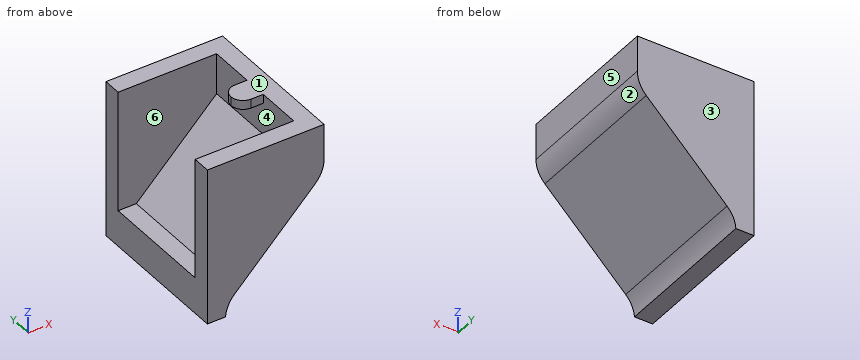
```python
from build123d import *

# Parameters (mm, degrees)
SKETCH_1_W          = 10
SKETCH_1_H          = 15
EXTRUDE_1_DEPTH     = 3
SKETCH_2_W          = 3
SKETCH_2_H          = 25
EXTRUDE_2_DEPTH     = 6
EXTRUDE_3_DEPTH     = 25
EXTRUDE_4_DEPTH     = 3
EXTRUDE_5_DEPTH     = 3
FILLET_1_R          = 5
SKETCH_6_W          = 10
SKETCH_6_H          = 15
CUT_EXTRUDE_1_DEPTH = 3
FILLET_2_R          = 5
SKETCH_7_W          = 1.5
SKETCH_7_H          = 4
EXTRUDE_6_DEPTH     = 4
FILLET_3_R          = 2


# Some blends are built 0.0001 mm under size
with BuildPart() as part:
    # 草图1 → 凸台-拉伸1 (new body)
    with BuildSketch(Plane.XY):
        with Locations((5, -7.5)):
            Rectangle(SKETCH_1_W, SKETCH_1_H)
    extrude(amount=EXTRUDE_1_DEPTH)

    # 草图2 → 凸台-拉伸2 (add)
    with BuildSketch(Plane.XY.offset(3)):
        with Locations((8.5, -7.5)):
            Rectangle(SKETCH_2_W, SKETCH_2_H)
    extrude(amount=EXTRUDE_2_DEPTH)

    # 草图3 → 凸台-拉伸3 (add)
    with BuildSketch(Plane(origin=(0, -20, 0), x_dir=(-1, 0, 0), z_dir=(0, -1, 0))):
        Polygon((-10, -9), (-23.263455967, -22.263455967), (-23.263455967, -29.02081528), (-26.263455967, -29.02081528), (-26.263455967, -21.02081528), (-10, -4.757359313), align=None)
    extrude(amount=-EXTRUDE_3_DEPTH)

    # 草图4 → 凸台-拉伸4 (add)
    with BuildSketch(Plane(origin=(0, -20, 0), x_dir=(-1, 0, 0), z_dir=(0, -1, 0))):
        Polygon((-7, -9), (-10, -9), (-23.263455967, -22.263455967), (-23.263455967, -29.02081528), (-7, -29.02081528), align=None)
    extrude(amount=-EXTRUDE_4_DEPTH)

    # 草图5 → 凸台-拉伸5 (add)
    with BuildSketch(Plane(origin=(0, 5, 0), x_dir=(1, 0, 0), z_dir=(0, 1, 0))):
        Polygon((7, -9), (10, -9), (23.263455967, -22.263455967), (23.263455967, -29.02081528), (7, -29.02081528), align=None)
    extrude(amount=-EXTRUDE_5_DEPTH)

    # 圆角1
    fillet_1_edges = [part.edges().sort_by_distance(p)[0] for p in [
        (26.263455967, -7.5, 21.02081528),
    ]]
    fillet(fillet_1_edges, radius=FILLET_1_R)

    # 草图6 → 切除-拉伸1 (cut)
    with BuildSketch(Plane(origin=(0, 0, 0), x_dir=(-1, 0, 0), z_dir=(0, 0, -1))):
        with Locations((-5, -7.5)):
            Rectangle(SKETCH_6_W, SKETCH_6_H)
    extrude(amount=-CUT_EXTRUDE_1_DEPTH, mode=Mode.SUBTRACT)

    # 圆角2
    # the kernel refuses this fillet: 5 mm, written as the material it adds along each edge
    with BuildSketch(Plane(origin=(10, -20, 4.757359313), x_dir=(0, 0, -1), z_dir=(0, 1, 0))) as fillet_2_piece_1:
        with BuildLine():
            CenterArc((2.08159154, -4.989476271), FILLET_2_R, 93.718036518, 41.281963482)
            Line((-1.453942365, -1.453942365), (-1.524653044, -1.383231687))
            Line((-1.524653044, -1.383231687), (-0.070710678, 0.070710678))
            Line((-0.070710678, 0.070710678), (0, 0.1))
            ThreePointArc((0, 0.1), (0.878679656, 0.1), (1.750874668, 0.099789525))
            Line((1.750874668, 0.099789525), (1.757359313, 0))
        make_face()
    extrude(amount=25)

    # 草图7 → 凸台-拉伸6 (add)
    with BuildSketch(Plane.ZY.offset(-23.263455967)):
        with Locations((28.27081528, -7.5)):
            Rectangle(SKETCH_7_W, SKETCH_7_H)
    extrude(amount=EXTRUDE_6_DEPTH)

    # 圆角3
    fillet_3_edges = [part.edges().sort_by_distance(p)[0] for p in [
        (19.263455967, -9.5, 28.27081528),
        (19.263455967, -5.5, 28.27081528),
    ]]
    fillet(fillet_3_edges, radius=FILLET_3_R - 0.0001)  # a hair under: the kernel refuses the full size


solid = part.part
```
Read the model definition and answer for the solid it produces. Units are mm, in the model's axes. Face numbers are marked on the shaded views. A direction names the side the tool comes from. Give positions to 0.01 mm unless a question says otherwise; leave off trailing zeros. Order: outer loops, then holes, each group sorted by start corner. A loop starts at its lowest first (then second) coordinate and runs counter-clockwise, first axis right, second up. Notation, with made-up numbers: (65, 50) -> (81, 50) arc R32 cw to (81, 77) -> close; hole circle Ø3 at (-39, -29.75). An arc over 180 degrees is marked (long way). Write item = value, one per line.
1. A cutting plane is placed at A-A, the plane x = 9. Write down the section's boundary in (y, z).
Numbers:
outline = (-20, 3) -> (5, 3) -> (5, 29.02) -> (2, 29.02) -> (2, 9) -> (-17, 9) -> (-17, 29.02) -> (-20, 29.02) -> close
2. For the marked faces 5 and 6, determine the directions among +Z, -Z, +X, -X, +Y, -Y from which every point of the face is accessible in a straight line to the end or side of a thin tool.
Numbers:
face_5 = +Z, -Z, +X, +Y, -Y
face_6 = +Z, -X
3. Straight lines are drawn through the part: line 1 along Y through (x, z) = (18.75, 20.75); line 2 along X through (y, z) = (-11.75, 27); line 3 along X through (y, z) = (-15, 20.5). For each, find the intervals that lie inside material, in ascending order.
Numbers:
line_1 = -20 to -17, 2 to 5
line_2 = 23.26 to 26.26
line_3 = 21.5 to 25.54
4. A cutting plane is placed at D-D, the plane z = 18.5. Write down the section's boundary in (x, y).
Numbers:
outline = (7, -20) -> (23.74, -20) -> (23.74, 5) -> (7, 5) -> (7, 2) -> (19.5, 2) -> (19.5, -17) -> (7, -17) -> close
5. A cutting plane is placed at C-C, the plane x = 22.5. Write down the section's boundary in (y, z).
Numbers:
outline = (-20, 17.26) -> (5, 17.26) -> (5, 29.02) -> (2, 29.02) -> (2, 21.5) -> (-17, 21.5) -> (-17, 29.02) -> (-20, 29.02) -> close; (-9.5, 27.52) -> (-5.5, 27.52) -> (-5.5, 29.02) -> (-9.5, 29.02) -> close
6. A cutting plane is placed at B-B, the plane y = -10. Write down the section's boundary in (x, z).
Numbers:
outline = (7, 3) -> (10, 3) arc R5 cw to (11.45, 6.21) -> (24.8, 19.56) arc R5 ccw to (26.26, 23.09) -> (26.26, 29.02) -> (23.26, 29.02) -> (23.26, 22.26) -> (10, 9) -> (7, 9) -> close
7. Given pin 1 (2 mm diameter, centred on x = 21.5, y = -7, fed in from -Z); pin 2 (10 mm diameter, centred on y = 1.5, z = 18, fed in from -X); pin 3 (0.9 mm diameter, centred on x = 8.5, y = -8.5, fed in from +Z), each flat-ended and moving along its own axis, determine where each tip first touches the part or whether it passes through.
Numbers:
pin_1 = 15.26
pin_2 = 7
pin_3 = 9
8. The mould has two halves that part along Z. Classify the marked faces 1, 2, 3 and 4: +Z half, -Z half, draft (parallel to the pull), parting line (faces both ways), or undercut.
Numbers:
face_1 = +Z half
face_2 = -Z half
face_3 = draft
face_4 = undercut
